Autodesk Inventor part; units mm, degrees
ref_plane "bolt_XY" through (0, 0, 0) normal (1, 0, 0) x (0, 0, -1)
ref_plane "bolt_YZ" through (0, 0, 0) normal (0, 0, -1) x (0, 1, 0)
ref_plane "bolt_ZX" through (0, 0, 0) normal (0, 1, 0) x (1, 0, 0)
sketch "Sketch_1" plane through (0, 0, 0) normal (0, 0, 1) x (1, 0, 0)
  line L0 (15, 0) -> (-4, 0)
  line L1 (-4, 0) -> (-4, 3.5)
  line L2 (-4, 3.5) -> (0, 3.5)
  line L3 (0, 3.5) -> (0, 2)
  line L4 (0, 2) -> (14.5705, 2)
  line L5 (14.5705, 2) -> (15, 1.5705)
  line L6 (15, 1.5705) -> (15, 0)
  line L7 (15, 0) -> (-4, 0)
revolve "Revolution1" add sketch "Sketch_1" angle 360 about axis through (15, 0, 0) along (1, 0, 0)
thread "Thread1"
sketch "Sketch_4" plane through (0, 0, 0) normal (0, 0, 1) x (1, 0, 0)
  line L0 (-1.5981, 0) -> (-4, 0)
  line L1 (-4, 0) -> (-4, 1.5)
  line L2 (-4, 1.5) -> (-2, 1.5)
  line L3 (-2, 1.5) -> (-1.5981, 0)
  line L4 (-1.5981, 0) -> (-4, 0)
revolve "Revolution2" cut sketch "Sketch_4" angle 360 about axis through (-1.5981, 0, 0) along (1, 0, 0)
sketch "Sketch_3" plane through (-4, 0, 0) normal (1, 0, 0) x (0, 0, -1)
  line L0 (-1.5, 0.866) -> (-1.5, -0.866)
  line L1 (-1.5, -0.866) -> (0, -1.7321)
  line L2 (0, -1.7321) -> (1.5, -0.866)
  line L3 (1.5, -0.866) -> (1.5, 0.866)
  line L4 (1.5, 0.866) -> (0, 1.7321)
  line L5 (0, 1.7321) -> (-1.5, 0.866)
extrude "Extrusion1" cut sketch "Sketch_3" along normal blind 2
ref_plane "bolt_XY" through (0, 0, 0) normal (1, 0, 0) x (0, 0, -1)
ref_plane "bolt_YZ" through (0, 0, 0) normal (0, 0, -1) x (0, 1, 0)
ref_plane "bolt_ZX" through (0, 0, 0) normal (0, 1, 0) x (1, 0, 0)
ref_plane "nut_XY" through (15, 0, 0) normal (1, 0, 0) x (0, 0, -1)
ref_plane "nut_YZ" through (15, 0, 0) normal (0, 0, -1) x (0, 1, 0)
ref_plane "nut_ZX" through (15, 0, 0) normal (0, 1, 0) x (1, 0, 0)
properties part number "CBM4-15" material "MISUMI"
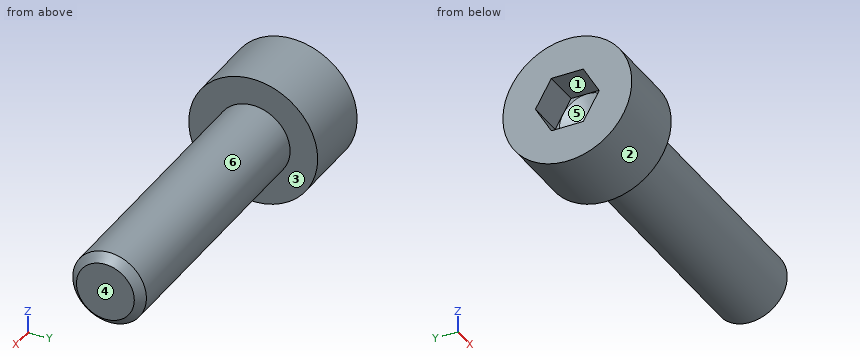
Build history of the part. All positions in model axes, mm. Face numbers are marked on the shaded views. A direction names the side the tool comes from. Coordinates: 2 decimals unless noted, no trailing zeros. Order: outer loops, then holes, each group sorted by start corner. A loop starts at its lowest first (then second) coordinate and runs counter-clockwise, first axis right, second up. Notation, with made-up numbers: (-11.5, 43.25) - (29.5, 43.25) arc R24 cw to (29.5, 73.25) - close; hole circle Ø3 at (-5.5, -14). An arc over 180 degrees is marked (long way). Write each question's results on one line, items separated by ' | '. Start each with the question number.
Item 1: Band-saw the part on A-A on x = 3.5. Write the cut outline in (y, z).
Item 2: Band-saw the part on D-D on x = -1. Write the cut outline in (y, z).
Item 3: Flat gauge pins, fed straight in: pin 1 (0.5 mm diameter, centred on x = -3, y = -0.5, fed in from +Z); pin 2 (1 mm diameter, centred on x = 6.5, y = -1, fed in from -Z); pin 3 (1.5 mm diameter, centred on x = 1, z = -2, fed in from -Y). Where does each tip first touch, or does it go through?
Item 4: Band-saw the part on B-B on y = 2.5. Write the cut outline in (x, z).
Item 5: Wall check: probe 1 along Y at (x, z) = (2.75, 1); probe 2 along X at (y, z) = (1, 3); probe 3 along Z at (x, y) = (6, 0). Give the ranges that are in metal, low to high. Write a range as [from, to].
Item 6: Mould opens along Y. For the marked faces 4, 5 and 6 say: released by +Y, released by -Y, zero draft, split by the parting line, or undercut.
Item 7: Tool access for the marked faces 1, 2 and 3: list every direction of +Z, -Z, +X, -X, +Y, -Y with a clear straight run to the whole face (end or side of a thin tool).
Item 8: Band-saw the part on C-C on z = 2.25. Write the cut outline in (x, y).
Numbers:
1) outline: circle Ø4 at (0, 0)
2) outline: circle Ø7 at (0, 0)
3) pin 1: z = 3.49 | pin 2: z = -1.94 | pin 3: y = -1.56
4) outline: (-4, -2.45) - (0, -2.45) - (0, 2.45) - (-4, 2.45) - close
5) probe 1: [-1.73, 1.73] | probe 2: [-4, 0] | probe 3: [-2, 2]
6) face 4: zero draft | face 5: undercut | face 6: split by the parting line
7) face 1: -X | face 2: +X, -X | face 3: +X
8) outline: (-4, -2.68) - (0, -2.68) - (0, 2.68) - (-4, 2.68) - close
